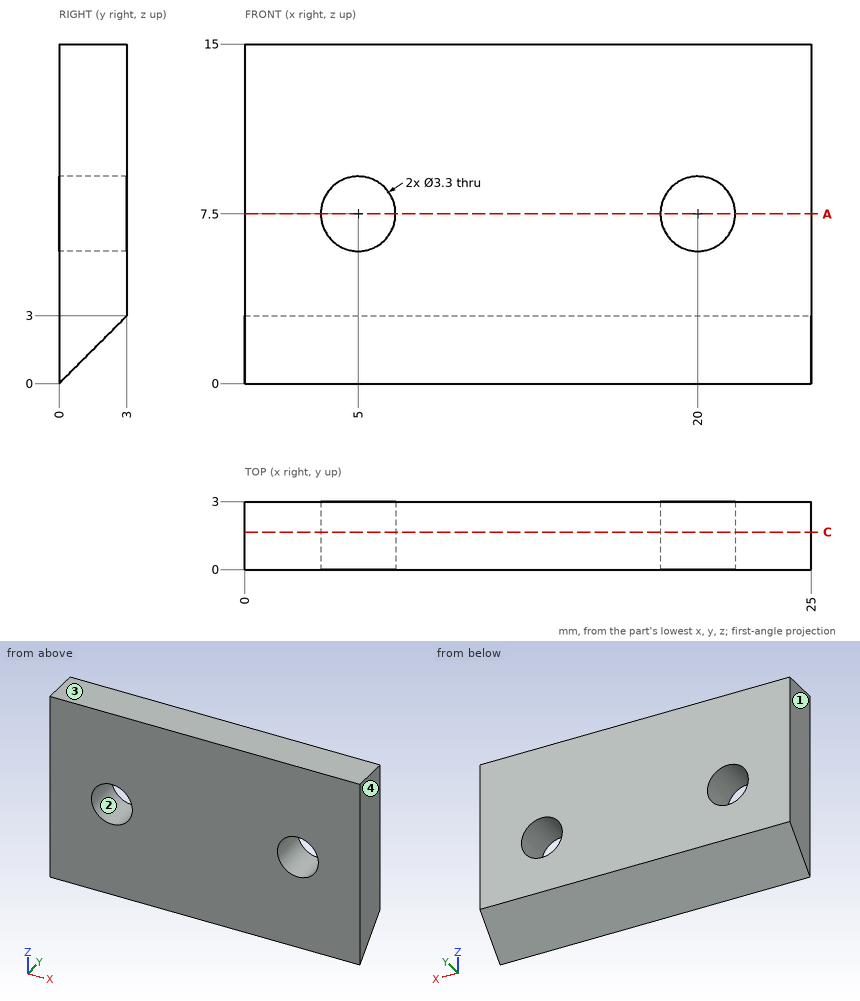
Geometry check sheet. Reference: drawing and pictorial views, mm from the part's lowest x, y, z. Round coordinates to 2 decimals unless told otherwise and drop trailing zeros. Write each loop counter-clockwise with the first axis right and the second up, starting at its lowest first coordinate (ties: lowest second). Pieces come first, ordered by that corner, then holes.
(1) Mould release check, pull along X, two halves, no side actions. Record for the marked faces 1, 2, 3 and 4: pulls with the +X half, pulls with the -X half, needs draft (parallel to the pull), parting line crosses it, or undercut.
Returned:
face 1: pulls with the -X half
face 2: undercut
face 3: needs draft
face 4: pulls with the +X half
(2) Section check C-C (y = 1.65). Enter the section's corners in (x, z).
Returned:
outline: (0, 1.65) - (25, 1.65) - (25, 15) - (0, 15) - close; hole circle Ø3.3 at (5, 7.5); hole circle Ø3.3 at (20, 7.5)
(3) Material ranges on line 1 (X direction, y = 0.75, z = 7.5); line 2 (X direction, y = 2.2, z = 6.25); line 3 (Z direction, x = 18.5, y = 0.55), recorded low to high.
Returned:
line 1: x = 0 to 3.35, 6.65 to 18.35, 21.65 to 25
line 2: x = 0 to 3.92, 6.08 to 18.92, 21.08 to 25
line 3: z = 0.55 to 6.81, 8.19 to 15
(4) Section check A-A (z = 7.5). Enter the section's corners in (x, y), plus the area to 3 significant figures.
Returned:
outline: (0, 0) - (3.35, 0) - (3.35, 3) - (0, 3) - close; (6.65, 0) - (18.35, 0) - (18.35, 3) - (6.65, 3) - close; (21.65, 0) - (25, 0) - (25, 3) - (21.65, 3) - close
area: 55.2 mm2
